Model file for the job. Use its own axes, mm. A direction names the side the tool comes from. Coordinates: 2 decimals unless noted, no trailing zeros. Write each loop counter-clockwise with the first axis right and the second up, starting at its lowest first coordinate (ties: lowest second). Pieces come first, ordered by that corner, then holes. Notation, with made-up numbers: (82, 40.25) -> (125, 40.25) arc R11 ccw to (125, 51.25) -> close; hole circle Ø8 at (-35, 12.5). An arc over 180 degrees is marked (long way). Write item = value, one per line. Start each with the question number.
from build123d import *

# Parameters (mm, degrees)
F0_W     = 40
F0_H     = 43
F0_W_2   = 36
F0_H_2   = 39
F1_DEPTH = 1.5
F2_DEPTH = 6
F3_W     = 2
F3_H     = 38
F4_DEPTH = 3.5
F5_R     = 2.5
F6_W     = 19
F6_H     = 1.3
F7_DEPTH = 5
F8_DEPTH = 1


with BuildPart() as f1:
    # F0 (on Top) → F1 (new body)
    with BuildSketch(Plane.XY):
        Rectangle(F0_W, F0_H)
        Rectangle(F0_W_2, F0_H_2, mode=Mode.SUBTRACT)
        Rectangle(F0_W_2, F0_H_2)
    extrude(amount=F1_DEPTH)

    # F0 (on Top) → F2 (join)
    with BuildSketch(Plane.XY):
        Rectangle(F0_W, F0_H)
        Rectangle(F0_W_2, F0_H_2, mode=Mode.SUBTRACT)
    extrude(amount=F2_DEPTH)

    # F3 (on face) → F4 (cut)
    with BuildSketch(Plane.XY.offset(6)):
        with Locations((-19, 0)):
            Rectangle(F3_W, F3_H)
    extrude(amount=-F4_DEPTH, mode=Mode.SUBTRACT)

    # F5
    f5_edges = [f1.edges().sort_by_distance(p)[0] for p in [
        (-20, -21.5, 3),
        (20, -21.5, 3),
        (20, 21.5, 3),
        (-20, 21.5, 3),
        (0, -21.5, 0),
        (20, 0, 0),
        (0, 21.5, 0),
    ]]
    fillet(f5_edges, radius=F5_R)

    # F6 (on face) → F7 (join)
    with BuildSketch(Plane.XY.offset(6)):
        with Locations((0, 20.2)):
            Rectangle(F6_W, F6_H)
        with Locations((0, -20.2)):
            Rectangle(F6_W, F6_H)
    extrude(amount=F7_DEPTH)

    # F3 (on face) → F8 (cut)
    with BuildSketch(Plane.XY.offset(6)):
        with Locations((19, 0)):
            Rectangle(F3_W, F3_H)
    extrude(amount=-F8_DEPTH, mode=Mode.SUBTRACT)


solid = f1.part
(1) Saw through at A-A (z = 8.25). Give the cut face in (x, y).
(2) Drop flat-ended pins along their axis: pin 1 Ø1 at (x, z) = (-18.5, 4.5) entering from -Y; pin 2 Ø0.6 at (x, z) = (-19.5, 5) entering from +Y; pin 3 Ø5.5 at (x, z) = (-3, 9.5) entering from -Y; pin 4 Ø5 at (y, z) = (-10.5, 9) entering from +X. Give the stop position or say it passes through.
(3) Saw through at B-B (x = -2). Give the cut face in (y, z), then the cut area to 3 significant figures.
(4) Drill centre lines: line 1 along Y through (x, z) = (9, 5.25); line 2 along Y through (x, z) = (1, 6.5); line 3 along Z through (x, y) = (-14.5, 18). Where is each one in solid material? Low to high.
(5) Saw through at C-C (y = -6). Give the cut face in (x, z).
(6) 3-axis set-ups, long thin cutter, end or side, ignore diameter. For faces 4 (the face through (0, -20.85, 8)), 5 (the face through (19, 19, 5.5)), 6 (the face through (-9.5, -20, 8)), 7 (the face through (9.5, -20, 8)): which of +Z, -Z, +X, -X, +Y, -Y reach the whole face in a straight line?
(7) Mould opens along X. For faces 1 (the face through (-18, 0, 2)), 2 (the face through (-20, 0, 1)), 3 (the face through (-1, -21, 1)) say: released by +X, released by -X, zero draft, split by the parting line, or undercut.
(8) Saw through at D-D (z = 3.25). Give the cut face in (x, y), then the cut area to 3 significant figures.
Returned:
q1.outline = (-9.5, -20.85) -> (9.5, -20.85) -> (9.5, -19.55) -> (-9.5, -19.55) -> close; (-9.5, 19.55) -> (9.5, 19.55) -> (9.5, 20.85) -> (-9.5, 20.85) -> close
q2.pin_1 = -21.45
q2.pin_2 = 20.83
q2.pin_3 = -20.85
q2.pin_4 = through
q3.outline = (-21.5, 2.5) arc R2.5 ccw to (-19, 0) -> (19, 0) arc R2.5 ccw to (21.5, 2.5) -> (21.5, 6) -> (20.85, 6) -> (20.85, 11) -> (19.55, 11) -> (19.55, 6) -> (19.5, 6) -> (19.5, 1.5) -> (-19.5, 1.5) -> (-19.5, 6) -> (-19.55, 6) -> (-19.55, 11) -> (-20.85, 11) -> (-20.85, 6) -> (-21.5, 6) -> close
q3.area = 92.8 mm2
q4.line_1 = -21.5 to -19.5, 19.5 to 21.5
q4.line_2 = -20.85 to -19.55, 19.55 to 20.85
q4.line_3 = 0 to 1.5
q5.outline = (-20, 0) -> (17.5, 0) arc R2.5 ccw to (20, 2.5) -> (20, 5) -> (18, 5) -> (18, 1.5) -> (-18, 1.5) -> (-18, 2.5) -> (-20, 2.5) -> close
q6.face_4 = +Z, +X, -X, -Y
q6.face_5 = +Z, +X, -X
q6.face_6 = +Z, -X, +Y, -Y
q6.face_7 = +Z, +X, +Y, -Y
q7.face_1 = undercut
q7.face_2 = released by -X
q7.face_3 = zero draft
q8.outline = (-20, -19) arc R2.5 ccw to (-17.5, -21.5) -> (17.5, -21.5) arc R2.5 ccw to (20, -19) -> (20, 19) arc R2.5 ccw to (17.5, 21.5) -> (-17.5, 21.5) arc R2.5 ccw to (-20, 19) -> (-18, 19) -> (-18, 19.5) -> (18, 19.5) -> (18, -19.5) -> (-18, -19.5) -> (-18, -19) -> close
q8.area = 235 mm2
